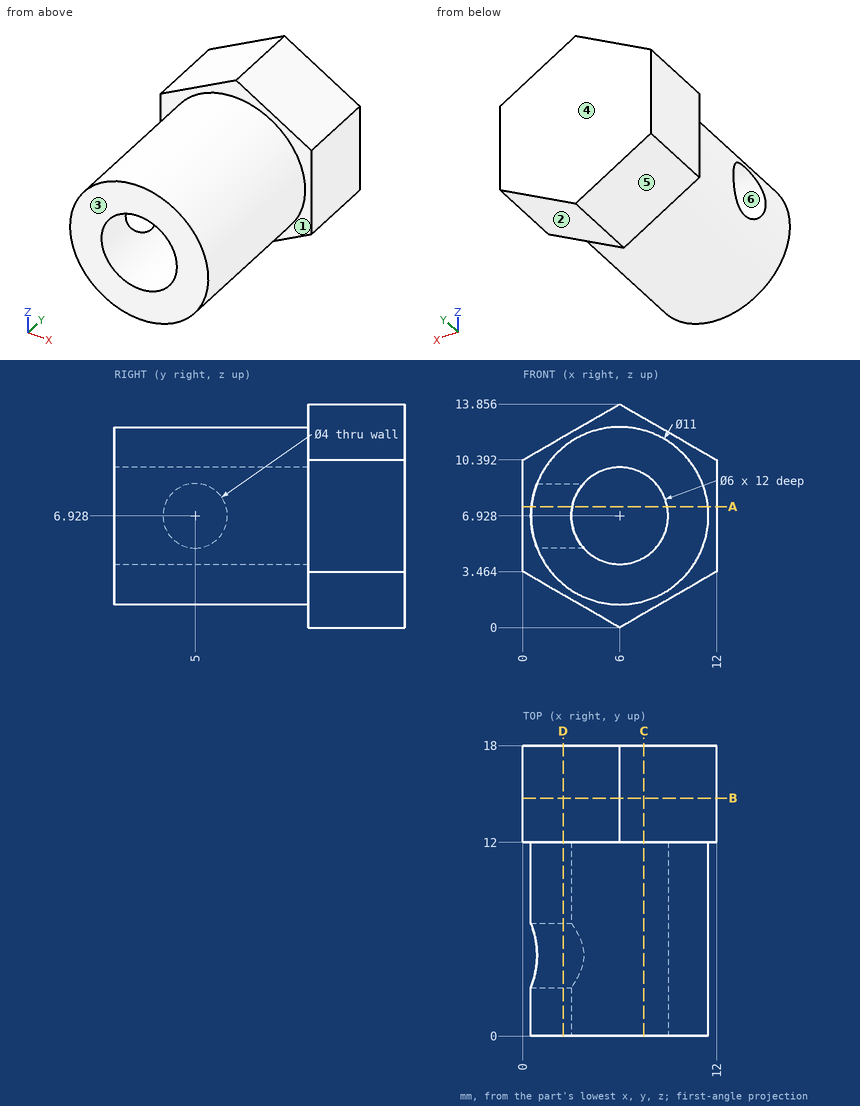
Input: dimensioned drawing with shaded views. Units: mm. Origin: part minimum x, y, z. A direction names the side the tool comes from. Give positions to 0.01 mm unless a question says otherwise; leave off trailing zeros. Write each loop counter-clockwise with the first axis right and the second up, starting at its lowest first coordinate (ties: lowest second). Pieces come first, ordered by that corner, then holes.
1. First-contact query: pin 1 (5 mm diameter, centred on x = 6, z = 6.93, fed in from -Y); pin 2 (3 mm diameter, centred on x = 2.5, y = 12.5, fed in from -Z) (1 decimal); pin 3 (4 mm diameter, centred on x = 6.5, y = 9.5, fed in from -Z). Flat tips, straight axial feed; report the tip coordinate or a pass-through.
2. Section query D-D (x = 2.5). Return the cut outline in (y, z) (1 decimal).
3. Section query A-A (z = 7.5). Return the cut outline in (x, y) (1 decimal).
4. Material intervals for line 1 along Y through (x, z) = (4.25, 12.5); line 2 along Z through (x, y) = (8.5, 1) (1 decimal); line 3 along Z through (x, y) = (4.5, 3.5) (1 decimal), sorted ascending.
5. Pull-direction query (Y, two-part tool) for the marked faces 3, 4, 5 and 6; classes: +Y half, -Y half, draft (parallel to the pull), parting line (faces both ways), or undercut.
6. Section query C-C (x = 7.5). Return the cut outline in (y, z).
7. Section query B-B (y = 14.75). Return the cut outline in (x, z).
8. Access query for the marked faces 1 and 2. Directions: +Z, -Z, +X, -X, +Y, -Y. A direction counts if a zero-diameter tool reaches every point of the face in a straight line with its end or side. Return the directions, or none.
Output values:
1. pin 1: stops at y = 12
1. pin 2: stops at z = 1.2
1. pin 3: stops at z = 1.43
2. outline: (0, 2.7) - (12, 2.7) - (12, 2) - (18, 2) - (18, 11.8) - (12, 11.8) - (12, 11.2) - (0, 11.2) - close; hole circle Ø4 at (5, 6.9)
3. outline: (0, 12) - (0.5, 12) - (0.5, 6.9) - (3.1, 6.9) - (3.1, 12) - (8.9, 12) - (8.9, 0) - (11.5, 0) - (11.5, 12) - (12, 12) - (12, 18) - (0, 18) - close; (0.5, 0) - (3.1, 0) - (3.1, 3.1) - (0.5, 3.1) - close
4. line 1: y = 12 to 18
4. line 2: z = 2 to 5.3, 8.6 to 11.8
4. line 3: z = 1.6 to 4.3, 9.5 to 12.2
5. face 3: -Y half
5. face 4: +Y half
5. face 5: draft
5. face 6: undercut
6. outline: (0, 1.64) - (12, 1.64) - (12, 0.87) - (18, 0.87) - (18, 12.99) - (12, 12.99) - (12, 12.22) - (0, 12.22) - (0, 9.53) - (12, 9.53) - (12, 4.33) - (0, 4.33) - close
7. outline: (0, 3.46) - (6, 0) - (12, 3.46) - (12, 10.39) - (6, 13.86) - (0, 10.39) - close
8. face 1: -Y
8. face 2: -Z, +X, +Y, -Y
